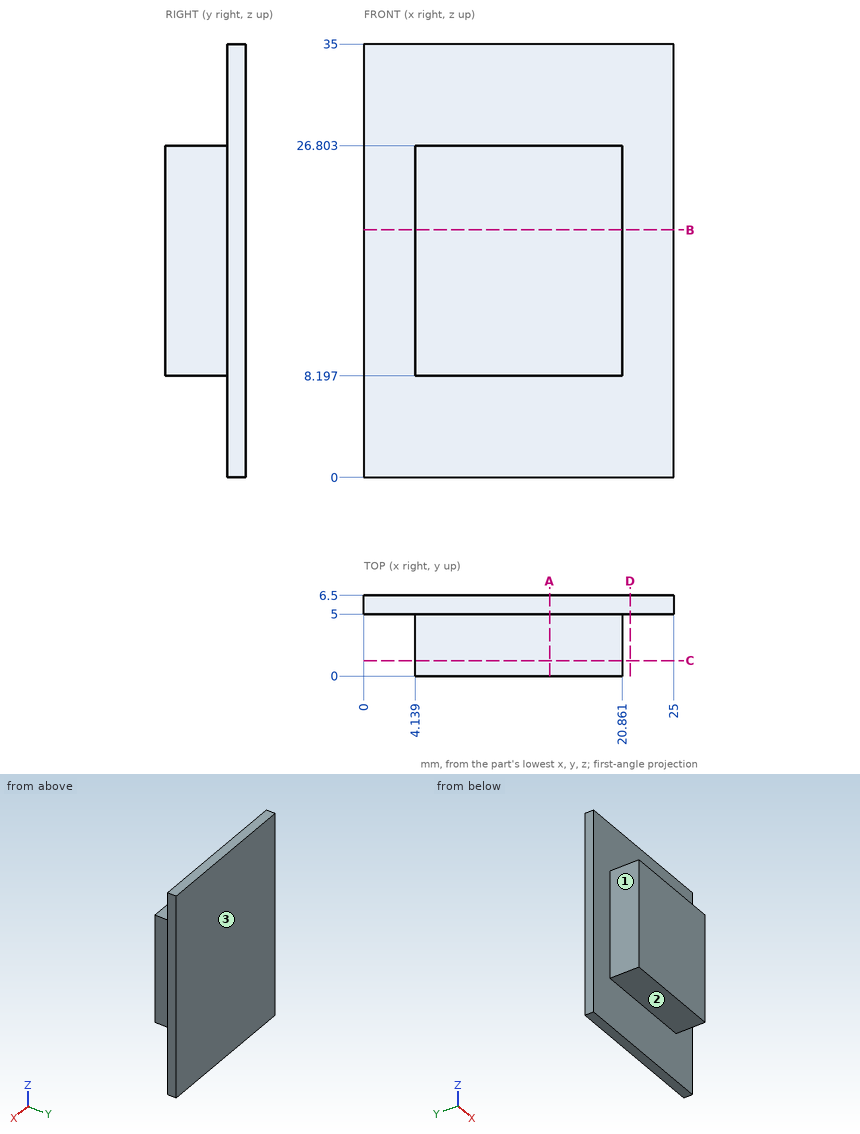
Verification items for this drawing (mm, ordinates from the low corner). A direction names the side the tool comes from. Give positions to 0.01 mm unless a question says otherwise; leave off trailing zeros. Order: outer loops, then holes, each group sorted by start corner. A loop starts at its lowest first (then second) coordinate and runs counter-clockwise, first axis right, second up. Notation, with made-up numbers: M 36,42.5 L 92,42.5 A23 cw 92,60.5 Z; hole C 53.25,8.25 d3. An arc over 180 degrees is marked long. Use a Markdown table: item, result.
Item 1: Section check C-C (y = 1.25). Record the cut outline in (x, z), and give its area (3 significant figures).
Answers follow:
| item | result |
|---|---|
| outline | M 4.14,8.2 L 20.86,8.2 L 20.86,26.8 L 4.14,26.8 Z |
| area | 311 mm2 |
Item 2: Section check A-A (x = 15). Record the cut outline in (y, z).
Answers follow:
| item | result |
|---|---|
| outline | M 0,8.2 L 5,8.2 L 5,0 L 6.5,0 L 6.5,35 L 5,35 L 5,26.8 L 0,26.8 Z |
Item 3: Depth check by flat-ended pin: P1, Ø2, axis at y = 1, z = 14, coming from the -X side; P2, Ø1.5, axis at y = 3.5, z = 19.5, coming from the +X side; P3, Ø1.5, axis at x = 7, y = 2.5, coming from the +Z side. Enter the tip coordinate at first touch or a pass-through.
Answers follow:
| item | result |
|---|---|
| P1 | stops at x = 4.14 |
| P2 | stops at x = 20.86 |
| P3 | stops at z = 26.8 |
Item 4: Material ranges on line 1 along Y through (x, z) = (1.5, 6); line 2 along Z through (x, y) = (8.75, 4.25); line 3 along X through (y, z) = (1.25, 12.5), recorded low to high.
Answers follow:
| item | result |
|---|---|
| line 1 | y = 5 to 6.5 |
| line 2 | z = 8.2 to 26.8 |
| line 3 | x = 4.14 to 20.86 |
Item 5: Tool access check on the marked faces 1, 2 and 3. Record the directions out of +Z, -Z, +X, -X, +Y, -Y that give a thin tool (end or side, any length) a straight path to the whole face; none if there is none.
Answers follow:
| item | result |
|---|---|
| face 1 | +Z, -Z, -X, -Y |
| face 2 | -Z, +X, -X, -Y |
| face 3 | +Z, -Z, +X, -X, +Y |
Item 6: Section check B-B (z = 20). Record the cut outline in (x, y).
Answers follow:
| item | result |
|---|---|
| outline | M 0,5 L 4.14,5 L 4.14,0 L 20.86,0 L 20.86,5 L 25,5 L 25,6.5 L 0,6.5 Z |
Item 7: Section check D-D (x = 21.5). Record the cut outline in (y, z), and give its area (3 significant figures).
Answers follow:
| item | result |
|---|---|
| outline | M 5,0 L 6.5,0 L 6.5,35 L 5,35 Z |
| area | 52.5 mm2 |
